Source: CAD feature listing. Evaluate the final solid. Frame: model axes, mm. Give positions to 0.01 mm unless a question says otherwise; leave off trailing zeros. Order: outer loops, then holes, each group sorted by start corner. A loop starts at its lowest first (then second) coordinate and runs counter-clockwise, first axis right, second up.
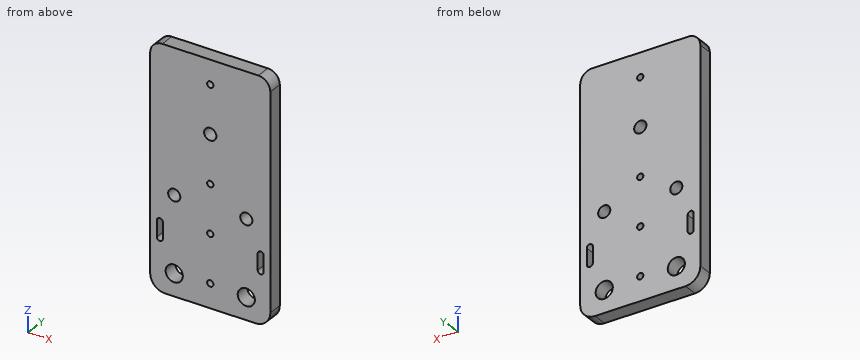
from build123d import *

# Parameters (mm, degrees)
F0_R     = 3.57
F0_R_2   = 2.525
F0_R_3   = 1.3
F0_R_4   = 2.55
F1_DEPTH = 6


with BuildPart() as f1:
    # F0 (on Front) → F1 (new body)
    with BuildSketch(Plane.XZ):
        with BuildLine():
            Line((20, 59.525), (18.83, 59.525))
            Line((18.83, 59.525), (-18.83, 59.525))
            Line((-18.83, 59.525), (-20, 59.525))
            ThreePointArc((-20, 59.525), (-23.535534, 58.060534), (-25, 54.525))
            Line((-25, 54.525), (-25, 50.695))
            Line((-25, 50.695), (-25, -34.305))
            ThreePointArc((-25, -34.305), (-23.192849, -38.667849), (-18.83, -40.475))
            Line((-18.83, -40.475), (18.83, -40.475))
            ThreePointArc((18.83, -40.475), (23.192849, -38.667849), (25, -34.305))
            Line((25, -34.305), (25, 50.695))
            Line((25, 50.695), (25, 54.525))
            ThreePointArc((25, 54.525), (23.535534, 58.060534), (20, 59.525))
        make_face()
        with Locations((-15, -31.225)):
            Circle(F0_R, mode=Mode.SUBTRACT)
        with BuildLine():
            Line((-19.755, -12.125), (-19.755, -18.825))
            ThreePointArc((-19.755, -18.825), (-21.005, -20.075), (-22.255, -18.825))
            Line((-22.255, -18.825), (-22.255, -12.125))
            ThreePointArc((-22.255, -12.125), (-21.005, -10.875), (-19.755, -12.125))
        make_face(mode=Mode.SUBTRACT)
        with Locations((-15, 0.275)):
            Circle(F0_R_2, mode=Mode.SUBTRACT)
        with Locations((0, -30.475)):
            Circle(F0_R_3, mode=Mode.SUBTRACT)
        with Locations((15, -31.225)):
            Circle(F0_R, mode=Mode.SUBTRACT)
        with Locations((0, -10.475)):
            Circle(F0_R_3, mode=Mode.SUBTRACT)
        with BuildLine():
            Line((22.255, -12.125), (22.255, -18.825))
            ThreePointArc((22.255, -18.825), (21.005, -20.075), (19.755, -18.825))
            Line((19.755, -18.825), (19.755, -12.125))
            ThreePointArc((19.755, -12.125), (21.005, -10.875), (22.255, -12.125))
        make_face(mode=Mode.SUBTRACT)
        with Locations((15, 0.275)):
            Circle(F0_R_2, mode=Mode.SUBTRACT)
        with Locations((0, 9.525)):
            Circle(F0_R_3, mode=Mode.SUBTRACT)
        with Locations((0, 29.525)):
            Circle(F0_R_4, mode=Mode.SUBTRACT)
        with Locations((0, 49.525)):
            Circle(F0_R_3, mode=Mode.SUBTRACT)
    extrude(amount=F1_DEPTH)


solid = f1.part
1) First-contact query: pin 1 Ø4 at (x, z) = (0, 29.525) entering from +Y. Flat tip, straight axial feed; report the tip coordinate or a pass-through.
Checks:
pin 1: passes through
2) Section query A-A on x = -15. Output: boundary loops of the cut face in (y, z) (3 decimals).
Checks:
outline: (-6, -40.475) - (0, -40.475) - (0, -34.795) - (-6, -34.795) - close; (-6, -27.655) - (0, -27.655) - (0, -2.25) - (-6, -2.25) - close; (-6, 2.8) - (0, 2.8) - (0, 59.525) - (-6, 59.525) - close
3) Section query B-B on y = -4.7. State how many separate pieces and enclosed holes the cut face has, and give its area (3 significant figures).
Checks:
separate pieces: 1
enclosed holes: 11
area: 4,770 mm2
4) Section query C-C on x = -21. Output: boundary loops of the cut face in (y, z), and give its area (3 significant figures).
Checks:
outline: (-6, -40.08) - (0, -40.08) - (0, -20.07) - (-6, -20.07) - close; (-6, -10.88) - (0, -10.88) - (0, 59.42) - (-6, 59.42) - close
area: 542 mm2
5) Ray query, L1, parallel to X at y = -4.2, z = -19; L2, parallel to Z at x = 0, y = -3.2 (3 decimals); L3, parallel to Z at x = 15, y = -4.1 (3 decimals). Return the intervals inside material, ascending.
Checks:
L1: x = -25 to -22.24, -19.77 to 19.77, 22.24 to 25
L2: z = -40.475 to -31.775, -29.175 to -11.775, -9.175 to 8.225, 10.825 to 26.975, 32.075 to 48.225, 50.825 to 59.525
L3: z = -40.475 to -34.795, -27.655 to -2.25, 2.8 to 59.525
